Read the model definition and answer for the solid it produces. Units are mm, in the model's axes. A direction names the side the tool comes from. Coordinates: 2 decimals unless noted, no trailing zeros. Order: outer loops, then holes, each group sorted by start corner. A loop starts at its lowest first (then second) coordinate and runs counter-clockwise, first axis right, second up. Notation, with made-up numbers: (-27, 1.25) -> (17, 1.25) arc R35 cw to (17, 37.25) -> close; hole circle Ø8 at (77.25, 4). An arc over 180 degrees is marked (long way). Use CSV: the item, a comma, the result in double quotes.
```python
from build123d import *

# Parameters (mm, degrees)
F1_DEPTH = 3
F2_R     = 5
F3_R     = 5
F4_R     = 10
F5_R     = 10


with BuildPart() as f1:
    # F0 (on Front) → F1 (new body)
    with BuildSketch(Plane.XZ):
        Polygon((-50, 0), (0, 0), (0, -12), (-15, -12), (-15, -22), (25, -22), (25, -12), (10, -12), (10, 0), (60, 0), (76.583124, 25), (-66.583124, 25), align=None)
    extrude(amount=F1_DEPTH)

    # F2
    f2_edges = [f1.edges().sort_by_distance(p)[0] for p in [
        (25, -1.5, -12),
    ]]
    fillet(f2_edges, radius=F2_R)

    # F3
    f3_edges = [f1.edges().sort_by_distance(p)[0] for p in [
        (-15, -1.5, -12),
    ]]
    fillet(f3_edges, radius=F3_R)

    # F4
    f4_edges = [f1.edges().sort_by_distance(p)[0] for p in [
        (60, -1.5, 0),
    ]]
    fillet(f4_edges, radius=F4_R)

    # F5
    f5_edges = [f1.edges().sort_by_distance(p)[0] for p in [
        (-50, -1.5, 0),
    ]]
    fillet(f5_edges, radius=F5_R)


solid = f1.part
```
Item 1: Find section D-D, the plane x = -40.5. Give the vertices of the cut face in (y, z).
Return value:
outline,"(-3, 0) -> (0, 0) -> (0, 25) -> (-3, 25) -> close"
Item 2: Straight lines are drawn through the part: line 1 along X through (y, z) = (-1.25, -6); line 2 along Z through (x, y) = (-18, -0.6); line 3 along Z through (x, y) = (15, -2.45). For each, find the intervals that lie inside material, in ascending order.
Return value:
line 1,"x = 0 to 10"
line 2,"z = 0 to 25"
line 3,"z = -22 to -12, 0 to 25"
Item 3: Find section C-C, the plane z = -10. Give the vertices of the cut face in (x, y), then the cut area to 3 significant figures.
Return value:
outline,"(0, -3) -> (10, -3) -> (10, 0) -> (0, 0) -> close"
area,"30.0 mm^2"
Item 4: Find section A-A, the plane x = -8. Give the vertices of the cut face in (y, z).
Return value:
outline,"(-3, -22) -> (0, -22) -> (0, -12) -> (-3, -12) -> close; (-3, 0) -> (0, 0) -> (0, 25) -> (-3, 25) -> close"
Item 5: Find section B-B, the plane y = -0.6. Give the vertices of the cut face in (x, z).
Return value:
outline,"(-66.58, 25) -> (-52.97, 4.47) arc R10 ccw to (-44.63, 0) -> (0, 0) -> (0, -12) -> (-10, -12) arc R5 ccw to (-15, -17) -> (-15, -22) -> (25, -22) -> (25, -17) arc R5 ccw to (20, -12) -> (10, -12) -> (10, 0) -> (54.63, 0) arc R10 ccw to (62.97, 4.47) -> (76.58, 25) -> close"
Item 6: The mould has two halves that part along Z. Classify faces 5 (the flat face through (15, -1, -12)), 6 (the flat face through (-15, -1, -19)), 7 (the cylindrical face through (59.301, -1.521, 1.156)): +Z half, -Z half, draft (parallel to the pull), parting line (faces both ways), or undercut.
Return value:
face 5,"undercut"
face 6,"draft"
face 7,"-Z half"
Item 7: Each of these flat-tipped pins is pushed along its axis until it touches: P1, Ø1, axis at y = -1, z = 10.5, coming from the +X side; P2, Ø1.5, axis at y = -2, z = -8.5, coming from the +X side; P3, Ø0.9, axis at y = -1.5, z = -19.5, coming from the +X side; P4, Ø10, axis at x = 34, z = -12, coming from the -Y side. Where does it stop, or does it pass through?
Return value:
P1,"stops at x = 67.3"
P2,"stops at x = 10"
P3,"stops at x = 25"
P4,"passes through"
Item 8: A tool of negligible diameter and unlimited length cuts with its end or side. For faces 1 (the cylindrical face through (-14, -2, -14)), 2 (the flat face through (32, -1, 0)), 3 (the flat face through (4, -3, 7)), 4 (the flat face through (25, -1, -20)), from which of +Z, -Z, +X, -X, +Y, -Y can it reach the whole face along a straight path? Write none if from no direction.
Return value:
face 1,"-X, +Y, -Y"
face 2,"+X, +Y, -Y"
face 3,"+Z, -Z, +X, -X, -Y"
face 4,"-Z, +X, +Y, -Y"
